Read the model definition and answer for the solid it produces. Units are mm, in the model's axes. Face numbers are marked on the shaded views. A direction names the side the tool comes from. Coordinates: 2 decimals unless noted, no trailing zeros. Order: outer loops, then holes, each group sorted by start corner. A loop starts at its lowest first (then second) coordinate and runs counter-clockwise, first axis right, second up. Notation, with made-up numbers: (23.5, 82) -> (42.5, 82) arc R11 cw to (42.5, 101) -> close; hole circle Ø7 at (34.25, 36.25). An arc over 180 degrees is marked (long way). Return JSON: item names as keys, results as strings. Group by question number.
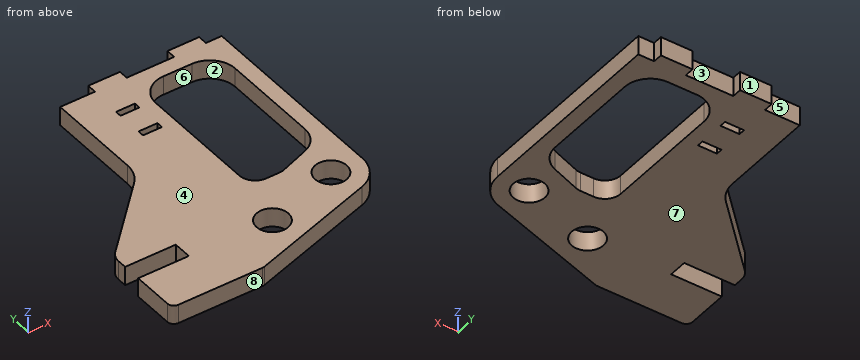
Autodesk Inventor part; units mm, degrees
ref_plane "YZ Plane" through (0, 0, 0) normal (1, 0, 0) x (0, 1, 0)
ref_plane "XZ Plane" through (0, 0, 0) normal (0, 1, 0) x (-1, 0, 0)
ref_plane "XY Plane" through (0, 0, 0) normal (0, 0, 1) x (1, 0, 0)
sketch "Sketch1" plane through (0, 0, 0) normal (0, 0, 1) x (1, 0, 0)
  line L0 (51, -62.5841) -> (51, 0)
  line L1 (21, 0) -> (21, 3)
  line L2 (21, 3) -> (11, 3)
  line L3 (11, 3) -> (11, 0)
  line L4 (36, 0) -> (36, 3)
  line L5 (36, 3) -> (46, 3)
  line L6 (46, 3) -> (46, 0)
  line L7 (51, 0) -> (46, 0)
  line L8 (36, 0) -> (21, 0)
  line L9 (11, 0) -> (0, 0)
  line L10 (-9, -69.8) -> (-25, -69.8)
  line L11 (-9, -64) -> (-25, -64)
  line L12 (-9, -69.8) -> (-9, -64)
  line L13 (-25, -69.8) -> (-25, -82.8)
  line L14 (29, -5) -> (38, -5)
  line L15 (46, -13) -> (46, -43.9388)
  line L16 (21, -50) -> (21, -13)
  arc A0 (29, -5) -> (21, -13) centre (29, -13) ccw
  arc A1 (46, -13) -> (38, -5) centre (38, -13) ccw
  line L17 (4.2384, -84.7068) -> (44.0172, -72.118)
  line L18 (26, -55) -> (30.1184, -55)
  line L19 (31.8285, -54.6985) -> (40.7362, -51.4563)
  arc A2 (21, -50) -> (26, -55) centre (26, -50) ccw
  arc A3 (30.1184, -55) -> (31.8285, -54.6985) centre (30.1184, -50) ccw
  arc A4 (40.7362, -51.4563) -> (46, -43.9388) centre (38, -43.9388) ccw
  arc A5 (44.0172, -72.118) -> (51, -62.5841) centre (41, -62.5841) ccw
  circle A6 centre (17.1651, -70.1271) radius 5
  circle A7 centre (41, -62.5841) radius 5
  line L20 (-25, -64) -> (-25, -61.0711)
  line L21 (-23.5355, -57.5355) -> (-2.9289, -36.9289)
  line L22 (0, -29.8579) -> (0, 0)
  arc A8 (-2.9289, -36.9289) -> (0, -29.8579) centre (-10, -29.8579) ccw
  arc A9 (-23.5355, -57.5355) -> (-25, -61.0711) centre (-20, -61.0711) ccw
  line L23 (-23, -84.8) -> (3.635, -84.8)
  arc A10 (-25, -82.8) -> (-23, -84.8) centre (-23, -82.8) ccw
  arc A11 (3.635, -84.8) -> (4.2384, -84.7068) centre (3.635, -82.8) ccw
  point P0 (0, 0)
  point P1 (16, 3)
  point P2 (41, 3)
  point P3 (51, -69.9082)
  point P4 (-25, -84.8)
  point P5 (46, -49.5404)
  point P6 (21, -55)
  point P7 (31, -55)
  point P8 (-25, -59)
  point P9 (0, -34)
  dimension "d17" = 10
  dimension "d18" = 3
  dimension "d20" = 10
  dimension "d21" = 3
  dimension "d22" = 5
  dimension "d23" = 15
  dimension "d24" = 3
  dimension "d25" = 3
  dimension "d75" = 90
  dimension "d129" = 64
  dimension "d130" = 16
  dimension "d131" = 60
  dimension "d139" = 5.8
  dimension "d148" = 5
  dimension "d149" = 5
  dimension "d152" = 8
  dimension "d162" = 10
  dimension "d164" = 160
  dimension "d167" = 55
  dimension "d169" = 5
  dimension "d170" = 5
  dimension "d171" = 8
  dimension "d173" = 10
  dimension "d184" = 5
  dimension "d185" = 30
  dimension "d186" = 135
  dimension "d187" = 10
  dimension "d188" = 5
  dimension "d189" = 25
  dimension "d190" = 15
  dimension "d191" = 25
  dimension "d192" = 2
extrude "Extrusion10" add sketch "Sketch1" along normal blind 6
sketch "Sketch3" plane through (0, 0, 0) normal (0, 0, -1) x (-1, 0, 0)
  line L0 (0, -29.8579) -> (0, 0) construction
  line L1 (-21, -50) -> (-21, -13) construction
  line L2 (-21, -13) -> (-21, -50) construction
  line L3 (0, 0) -> (-11, 0) construction
  line L4 (-10.5, -12) -> (-16.5, -12)
  line L5 (-16.5, -12) -> (-16.5, -10)
  line L6 (-16.5, -10) -> (-10.5, -10)
  line L7 (-10.5, -10) -> (-10.5, -12)
  line L8 (-10.5, -22) -> (-16.5, -22)
  line L9 (-16.5, -22) -> (-16.5, -20)
  line L10 (-16.5, -20) -> (-10.5, -20)
  line L11 (-10.5, -20) -> (-10.5, -22)
  point P0 (-13.5, -10)
  dimension "d204" = 2
  dimension "d205" = 6
  dimension "d206" = 8
  dimension "d207" = 4.5
extrude "Extrusion12" cut sketch "Sketch3" against normal through all
properties part number "Handle 27021014"
1. Find section B-B on y = -40. Determine the outline of the cut face in (x, z).
2. Given pin 1 (0.9 mm diameter, centred on y = 1, z = 4, fed in from -X); pin 2 (1.5 mm diameter, centred on x = 49, z = 3.5, fed in from +Y); pin 3 (2 mm diameter, centred on y = -14, z = 1.5, fed in from -X); pin 4 (16 mm diameter, centred on x = 17.17, y = -70.13, fed in from -Z), each flat-ended and moving along its own axis, determine where each tip first touches the part or whether it passes through.
3. For a pull along Y with two mould halves and no side action, classify the marked faces 6, 7 and 8 as released by +Y, released by -Y, zero draft, split by the parting line, or undercut.
4. Which of the six approach directions +Z, -Z, +X, -X, +Y, -Y give full straight-line access (tool end or side, diameter ignored) to the marked faces 1, 2, 3, 4 and 5?
5. Find section C-C on x = 2. Determine the outline of the cut face in (y, z), and give its area (3 significant figures).
6. Straight lines are drawn through the part: L1, parallel to Y at x = 41, z = 4.4; L2, parallel to Y at x = 15, z = 1.1; L3, parallel to X at y = -28, z = 4.5. For each, find the intervals that lie inside material, in ascending order.
7. Find section A-A on x = -14. Determine the outline of the cut face in (y, z).
8. Find section D-D on z = 5.05. Give the number of separate pieces and of enclosed holes in the cut face, and give its area (3 significant figures).
Result:
{
 "1": {"outline": "(-6, 0) -> (21, 0) -> (21, 6) -> (-6, 6) -> close; (46, 0) -> (51, 0) -> (51, 6) -> (46, 6) -> close"},
 "2": {"pin 1": "x = 11", "pin 2": "y = 0", "pin 3": "x = 0", "pin 4": "z = 0"},
 "3": {"face 6": "undercut", "face 7": "zero draft", "face 8": "released by -Y"},
 "4": {"face 1": "+Z, -Z, +X, -X, +Y", "face 2": "+Z, -Z", "face 3": "+Z, -Z, +Y", "face 4": "+Z, +X, -X, +Y, -Y", "face 5": "+Z, -Z, -X, +Y"},
 "5": {"outline": "(-84.8, 0) -> (0, 0) -> (0, 6) -> (-84.8, 6) -> close", "area": "509 mm^2"},
 "6": {"L1": "-73.07 to -67.58, -57.58 to -51.35, -5.58 to 3", "L2": "-81.3 to -74.63, -65.62 to -22, -20 to -12, -10 to 3", "L3": "0 to 21, 46 to 51"},
 "7": {"outline": "(-84.8, 0) -> (-69.8, 0) -> (-69.8, 6) -> (-84.8, 6) -> close; (-64, 0) -> (-48, 0) -> (-48, 6) -> (-64, 6) -> close"},
 "8": {"separate pieces": "1", "enclosed holes": "5", "area": "3,540 mm^2"}
}
